Read the model definition and answer for the solid it produces. Units are mm, in the model's axes. Face numbers are marked on the shaded views. A direction names the side the tool comes from. Coordinates: 2 decimals unless noted, no trailing zeros. Loops run counter-clockwise (first coordinate to the right, second up) from the corner with the lowest first, then second, coordinate; pieces in that order, holes last.
from build123d import *

# Parameters (mm, degrees)
SKETCH1_R           = 14.35
SKETCH1_R_2         = 5
BOSS_EXTRUDE1_DEPTH = 18
SKETCH2_R           = 20
BOSS_EXTRUDE2_DEPTH = 18
SKETCH3_R           = 16
BOSS_EXTRUDE3_DEPTH = 35.7
SKETCH5_OUTSIDE_W   = 123.14
SKETCH5_OUTSIDE_H   = 152.554
SKETCH5_OUTSIDE_R   = 14.935
CUT_EXTRUDE1_DEPTH  = 19
SKETCH7_R           = 4.25
CUT_EXTRUDE3_DEPTH  = 3
CUT_EXTRUDE3_DRAFT  = -38
SKETCH9_OUTSIDE_W   = 123.14
SKETCH9_OUTSIDE_H   = 152.554
SKETCH9_OUTSIDE_R   = 49.923055682
CUT_EXTRUDE4_DEPTH  = 1.35
SKETCH6_R           = 14.35
CUT_EXTRUDE5_DEPTH  = 21.7


with BuildPart() as part:
    # Sketch1 → Boss-Extrude1 (new body)
    with BuildSketch(Plane.XY):
        with BuildLine():
            Line((36.136520686, -18.774478422), (40.195752281, -43.049171521))
            ThreePointArc((40.195752281, -43.049171521), (0, -58.897620241), (-40.195752281, -43.049171521))
            Line((-40.195752281, -43.049171521), (-36.136520686, -18.774478422))
            ThreePointArc((-36.136520686, -18.774478422), (-36.697665198, -13.197066935), (-40.010085223, -8.674868838))
            ThreePointArc((-40.010085223, -8.674868838), (-44.039037615, 1.827589449), (-36.814887741, 10.449987378))
            ThreePointArc((-36.814887741, 10.449987378), (-32.208677837, 13.651878045), (-29.862109135, 18.747257211))
            Line((-29.862109135, 18.747257211), (-24.003146652, 53.784557457))
            ThreePointArc((-24.003146652, 53.784557457), (0, 58.897620241), (24.003146652, 53.784557457))
            Line((24.003146652, 53.784557457), (29.862109135, 18.747257211))
            ThreePointArc((29.862109135, 18.747257211), (32.208677837, 13.651878045), (36.814887741, 10.449987378))
            ThreePointArc((36.814887741, 10.449987378), (44.039037615, 1.827589449), (40.010085223, -8.674868838))
            ThreePointArc((40.010085223, -8.674868838), (36.697665198, -13.197066935), (36.136520686, -18.774478422))
        make_face()
        with Locations((0, 32.4)):
            Circle(SKETCH1_R, mode=Mode.SUBTRACT)
        with Locations((0.004379967, -44.949999787)):
            Circle(SKETCH1_R_2, mode=Mode.SUBTRACT)
    extrude(amount=-BOSS_EXTRUDE1_DEPTH)

    # Sketch2 → Boss-Extrude2 (add)
    with BuildSketch(Plane(origin=(0, 0, -18), x_dir=(-1, 0, 0), z_dir=(0, 0, -1))):
        with Locations(Location((0, 0, 0), (0, 0, 106.311047481))):
            Circle(SKETCH2_R)
    extrude(amount=BOSS_EXTRUDE2_DEPTH)

    # Sketch3 → Boss-Extrude3 (add)
    with BuildSketch(Plane(origin=(0, 0, -36), x_dir=(-1, 0, 0), z_dir=(0, 0, -1))):
        with Locations(Location((0, 0, 0), (0, 0, 180))):
            Circle(SKETCH3_R)
    extrude(amount=BOSS_EXTRUDE3_DEPTH)

    # Sketch5 outside → Cut-Extrude1 (cut)
    with BuildSketch(Plane(origin=(0, 0, -71.7), x_dir=(-1, 0, 0), z_dir=(0, 0, -1))):
        Rectangle(SKETCH5_OUTSIDE_W, SKETCH5_OUTSIDE_H)
        Circle(SKETCH5_OUTSIDE_R, mode=Mode.SUBTRACT)
    extrude(amount=-CUT_EXTRUDE1_DEPTH, mode=Mode.SUBTRACT)


with BuildPart() as cut_extrude3_tool:
    # Sketch7 → Cut-Extrude3 (with draft: the straight prism first)
    with BuildSketch(Plane.XY):
        Circle(SKETCH7_R)
    extrude(amount=-CUT_EXTRUDE3_DEPTH)
    # Cut-Extrude3: the draft: its side faces are tilted about the plane it starts from
    cut_extrude3_sides = [cut_extrude3_tool.faces().sort_by_distance(p)[0] for p in [
        (-4.25, 0, -1.5),
    ]]
    draft(cut_extrude3_sides, Plane.XY, CUT_EXTRUDE3_DRAFT)


with BuildPart() as part_1:
    add(part.part)

    # Cut-Extrude3: cut by cut_extrude3_tool
    add(cut_extrude3_tool.part, mode=Mode.SUBTRACT)

    # Sketch9 outside → Cut-Extrude4 (cut)
    with BuildSketch(Plane(origin=(0, 0, -18), x_dir=(-1, 0, 0), z_dir=(0, 0, -1))):
        Rectangle(SKETCH9_OUTSIDE_W, SKETCH9_OUTSIDE_H)
        Circle(SKETCH9_OUTSIDE_R, mode=Mode.SUBTRACT)
    extrude(amount=-CUT_EXTRUDE4_DEPTH, mode=Mode.SUBTRACT)

    # Sketch6 → Cut-Extrude5 (cut)
    with BuildSketch(Plane.XY):
        with Locations((0, 32.4)):
            Circle(SKETCH6_R)
    extrude(amount=-CUT_EXTRUDE5_DEPTH, mode=Mode.SUBTRACT)


solid = part_1.part
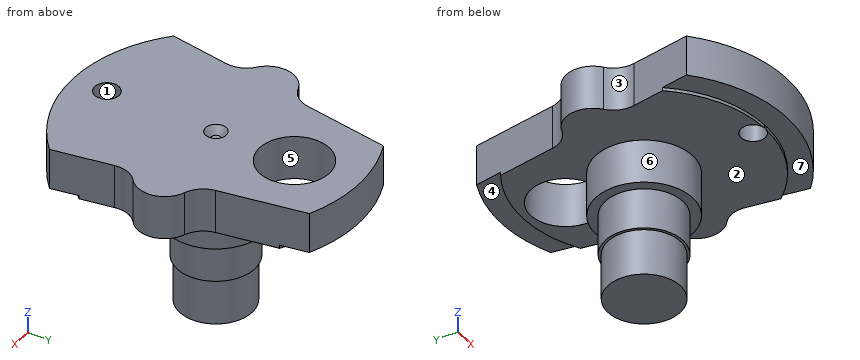
Item 1: Which of the six approach directions +Z, -Z, +X, -X, +Y, -Y give full straight-line access (tool end or side, diameter ignored) to the marked faces 4, 5, 6 and 7?
Numbers:
face 4: -Z, +Y
face 5: +Z
face 6: -Z
face 7: -Z, -Y
Item 2: Given pin 1 (1.1 mm diameter, centred on x = -0.5, y = 0.5, fed in from +Z); pin 2 (2 mm diameter, centred on y = 35, z = -11, fed in from +X); pin 3 (4 mm diameter, centred on x = -12.5, z = -29, fed in from +Y); pin 4 (1 mm diameter, centred on x = -22.5, y = 15, fed in from +Z), each flat-ended and moving along its own axis, determine where each tip first touches the part or whether it passes through.
Numbers:
pin 1: stops at z = -3
pin 2: stops at x = 27.31
pin 3: stops at y = 17.02
pin 4: stops at z = 0
Item 3: A cutting plane is placed at C-C on z = -56.5. Determine the outline of the cut face in (x, y) (3 decimals), then the cut area to 3 significant figures.
Numbers:
outline: circle Ø29.87 at (0, 0)
area: 701 mm2
Item 4: Determine the mould class of the marked faces 1, 2 and 3 for opening direction X: released by +X, released by -X, zero draft, split by the parting line, or undercut.
Numbers:
face 1: undercut
face 2: zero draft
face 3: released by -X
Item 5: A cutting plane is placed at B-B on x = 34.5. Determine the outline of the cut face in (y, z).
Numbers:
outline: (-47.74, -16.65) - (-36.08, -16.65) - (-36.08, -18) - (11.61, -18) - (11.61, 0) - (-47.74, 0) - close
Item 6: A cutting plane is placed at D-D on y = -44.95. Determine the outline of the cut face in (x, z).
Numbers:
outline: (-38.06, -16.65) - (-21.72, -16.65) - (-21.72, -18) - (-5, -18) - (-5, 0) - (-38.06, 0) - close; (5, -18) - (21.72, -18) - (21.72, -16.65) - (38.06, -16.65) - (38.06, 0) - (5, 0) - close
Item 7: A cutting plane is placed at A-A on y = 38. Determine the outline of the cut face in (x, z).
Numbers:
outline: (-26.64, -18) - (-13.21, -18) - (-13.21, 0) - (-26.64, 0) - close; (13.21, -18) - (26.64, -18) - (26.64, 0) - (13.21, 0) - close
Item 8: Find the intervals of material crossed by line 1 along Y through (x, z) = (0, -11.5); line 2 along Z through (x, y) = (-26, 29.5); line 3 along Z through (x, y) = (17.5, 4), in increasing order.
Numbers:
line 1: y = -58.9 to -49.95, -39.95 to 18.05, 46.75 to 58.9
line 2: z = -18 to 0
line 3: z = -36 to 0
